from build123d import *

# Parameters (mm, degrees)
ESBO_O1_W                = 300
ESBO_O1_H                = 180
ESBO_O1_R                = 1.5
ESBO_O1_R_2              = 2
ESBO_O1_R_3              = 15
ESBO_O1_R_4              = 4
ESBO_O1_R_5              = 1.65
ESBO_O1_R_6              = 1.75
ESBO_O1_W_2              = 20
ESBO_O1_H_2              = 20
RESSALTO_EXTRUS_O1_DEPTH = 6
ESBO_O2_R                = 2
CORTE_EXTRUS_O1_DEPTH    = 10


with BuildPart() as part:
    # Esboço1 → Ressalto-extrusão1 (new body)
    with BuildSketch(Plane.XY):
        Rectangle(ESBO_O1_W, ESBO_O1_H)
        with Locations((140, 45)):
            Circle(ESBO_O1_R, mode=Mode.SUBTRACT)
        with Locations((140, -40)):
            Circle(ESBO_O1_R, mode=Mode.SUBTRACT)
        with Locations((60, -40)):
            Circle(ESBO_O1_R, mode=Mode.SUBTRACT)
        with Locations((60, 45)):
            Circle(ESBO_O1_R, mode=Mode.SUBTRACT)
        with Locations((-107.5, -56.5)):
            Circle(ESBO_O1_R_2, mode=Mode.SUBTRACT)
        with Locations((-42.5, -56.5)):
            Circle(ESBO_O1_R_2, mode=Mode.SUBTRACT)
        with Locations((-75, -64)):
            Circle(ESBO_O1_R_3, mode=Mode.SUBTRACT)
        with Locations((-35, -64)):
            Circle(ESBO_O1_R_4, mode=Mode.SUBTRACT)
        with Locations((-115, -64)):
            Circle(ESBO_O1_R_4, mode=Mode.SUBTRACT)
        with Locations((-42.5, -71.5)):
            Circle(ESBO_O1_R_2, mode=Mode.SUBTRACT)
        with Locations((-107.5, -71.5)):
            Circle(ESBO_O1_R_2, mode=Mode.SUBTRACT)
        with Locations((35, 37)):
            Circle(ESBO_O1_R_5, mode=Mode.SUBTRACT)
        with Locations((35, 12)):
            Circle(ESBO_O1_R_5, mode=Mode.SUBTRACT)
        with Locations((-130, 60)):
            Circle(ESBO_O1_R_5, mode=Mode.SUBTRACT)
        with Locations((-20, 60)):
            Circle(ESBO_O1_R_5, mode=Mode.SUBTRACT)
        with Locations((-20, 5)):
            Circle(ESBO_O1_R_5, mode=Mode.SUBTRACT)
        with Locations((-130, 5)):
            Circle(ESBO_O1_R_5, mode=Mode.SUBTRACT)
        with Locations((95, -45)):
            Circle(ESBO_O1_R_6, mode=Mode.SUBTRACT)
        with Locations((95, -75)):
            Circle(ESBO_O1_R_6, mode=Mode.SUBTRACT)
        with Locations((100, -11.75)):
            Rectangle(ESBO_O1_W_2, ESBO_O1_H_2, mode=Mode.SUBTRACT)
    extrude(amount=RESSALTO_EXTRUS_O1_DEPTH)

    # Esboço2 → Corte-extrusão1 (cut)
    with BuildSketch(Plane.XY.offset(6)):
        with Locations((-140, 80)):
            Circle(ESBO_O2_R)
        with Locations((140, 80)):
            Circle(ESBO_O2_R)
        with Locations((120, -80)):
            Circle(ESBO_O2_R)
        with Locations((-140, -80)):
            Circle(ESBO_O2_R)
    extrude(amount=-CORTE_EXTRUS_O1_DEPTH, mode=Mode.SUBTRACT)


solid = part.part
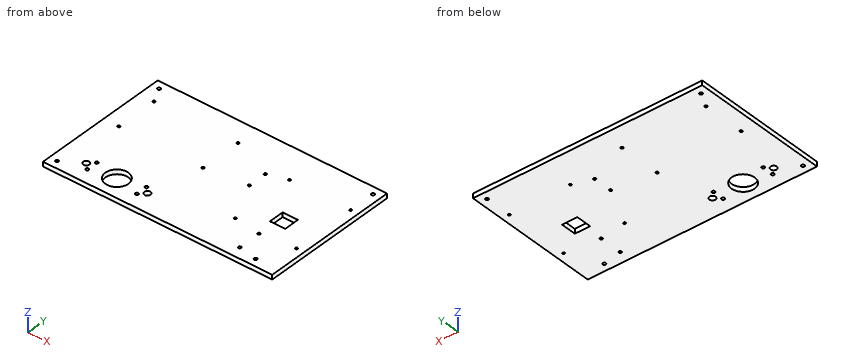
Geometry check sheet. Reference: the model listing, model coordinates, mm. Coordinates: 2 decimals unless noted, no trailing zeros. Order: outer loops, then holes, each group sorted by start corner. A loop starts at its lowest first (then second) coordinate and runs counter-clockwise, first axis right, second up. Notation, with made-up numbers: M 16,29 L 30,29 A10 cw 30,34 Z; hole C 7,21 d10. An arc over 180 degrees is marked long. Use CSV: the item, a comma, the result in double quotes.
Item 1: Cross-section at C-C on z = 1.35. Give the number of separate pieces and of enclosed holes in the cut face, then the cut area to 3 significant figures.
Returned:
separate pieces,"1"
enclosed holes,"24"
area,"52,600 mm2"
Item 2: Cross-section at B-B on x = -75. Record the cut outline in (y, z).
Returned:
outline,"M -90,0 L -79,0 L -79,6 L -90,6 Z; M -49,0 L 90,0 L 90,6 L -49,6 Z"
Item 3: Thickness scan on line 1 along Y through (x, z) = (-20, 2.3); line 2 along Y through (x, z) = (35, 2.95); line 3 along X through (y, z) = (-13, 1.8). Record the ranges inside material, lowest first.
Returned:
line 1,"y = -90 to 3.35, 6.65 to 58.35, 61.65 to 90"
line 2,"y = -90 to 10.35, 13.65 to 35.35, 38.65 to 90"
line 3,"x = -150 to 90, 110 to 150"
Item 4: Cross-section at A-A on y = -64. Record the cut outline in (x, z), then the cut area to 3 significant figures.
Returned:
outline,"M -150,0 L -119,0 L -119,6 L -150,6 Z; M -111,0 L -90,0 L -90,6 L -111,6 Z; M -60,0 L -39,0 L -39,6 L -60,6 Z; M -31,0 L 150,0 L 150,6 L -31,6 Z"
area,"1,520 mm2"
